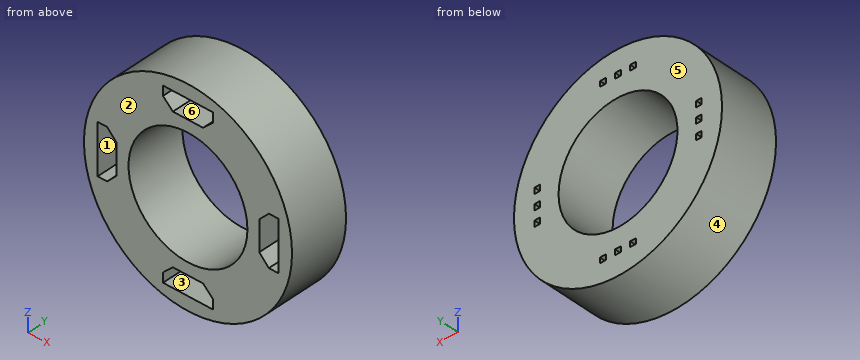
from build123d import *

# Parameters (mm, degrees)
F0_R     = 8.75
F0_R_2   = 5
F1_DEPTH = 5
F0_W     = 0.5
F0_H     = 0.45
F0_W_2   = 0.45
F0_H_2   = 0.5
F2_DEPTH = 1.5


with BuildPart() as f1:
    # F0 (on Front) → F1 (new body)
    with BuildSketch(Plane.XZ):
        Circle(F0_R)
        Polygon((-2.1, -6.8), (-1.27, -6), (1.27, -6), (2.1, -6.8), (2.1, -7.6), (-2.1, -7.6), align=None, mode=Mode.SUBTRACT)
        Polygon((-6.8, 2.1), (-6, 1.27), (-6, -1.27), (-6.8, -2.1), (-7.6, -2.1), (-7.6, 2.1), align=None, mode=Mode.SUBTRACT)
        Circle(F0_R_2, mode=Mode.SUBTRACT)
        Polygon((6.8, -2.1), (6, -1.27), (6, 1.27), (6.8, 2.1), (7.6, 2.1), (7.6, -2.1), align=None, mode=Mode.SUBTRACT)
        Polygon((-2.1, 6.8), (-2.1, 7.6), (2.1, 7.6), (2.1, 6.8), (1.27, 6), (-1.27, 6), align=None, mode=Mode.SUBTRACT)
    extrude(amount=F1_DEPTH)

    # F0 (on Front) → F2 (join)
    with BuildSketch(Plane.XZ):
        Polygon((2.1, 7.6), (-2.1, 7.6), (-2.1, 6.8), (-1.27, 6), (1.27, 6), (2.1, 6.8), align=None)
        with Locations((-1.27, 6.8)):
            Rectangle(F0_W, F0_H, mode=Mode.SUBTRACT)
        with Locations((0, 6.8)):
            Rectangle(F0_W, F0_H, mode=Mode.SUBTRACT)
        with Locations((1.27, 6.8)):
            Rectangle(F0_W, F0_H, mode=Mode.SUBTRACT)
        Polygon((-6, -1.27), (-6, 1.27), (-6.8, 2.1), (-7.6, 2.1), (-7.6, -2.1), (-6.8, -2.1), align=None)
        with Locations((-6.8, -1.27)):
            Rectangle(F0_W_2, F0_H_2, mode=Mode.SUBTRACT)
        with Locations((-6.8, 0)):
            Rectangle(F0_W_2, F0_H_2, mode=Mode.SUBTRACT)
        with Locations((-6.8, 1.27)):
            Rectangle(F0_W_2, F0_H_2, mode=Mode.SUBTRACT)
        Polygon((1.27, -6), (-1.27, -6), (-2.1, -6.8), (-2.1, -7.6), (2.1, -7.6), (2.1, -6.8), align=None)
        with Locations((-1.27, -6.8)):
            Rectangle(F0_W, F0_H, mode=Mode.SUBTRACT)
        with Locations((0, -6.8)):
            Rectangle(F0_W, F0_H, mode=Mode.SUBTRACT)
        with Locations((1.27, -6.8)):
            Rectangle(F0_W, F0_H, mode=Mode.SUBTRACT)
        Polygon((6, 1.27), (6, -1.27), (6.8, -2.1), (7.6, -2.1), (7.6, 2.1), (6.8, 2.1), align=None)
        with Locations((6.8, -1.27)):
            Rectangle(F0_W_2, F0_H_2, mode=Mode.SUBTRACT)
        with Locations((6.8, 0)):
            Rectangle(F0_W_2, F0_H_2, mode=Mode.SUBTRACT)
        with Locations((6.8, 1.27)):
            Rectangle(F0_W_2, F0_H_2, mode=Mode.SUBTRACT)
    extrude(amount=F2_DEPTH)


solid = f1.part
Check sheet for the modelled part. Datum: model origin and axes. Units: mm. Face numbers are marked on the shaded views. A direction names the side the tool comes from. Coordinates: 2 decimals unless noted, no trailing zeros. Loops run counter-clockwise (first coordinate to the right, second up) from the corner with the lowest first, then second, coordinate; pieces in that order, holes last. Notation, with made-up numbers: (77.5, 56.25) -> (125.5, 56.25) arc R22 cw to (125.5, 71.25) -> close; hole circle Ø9 at (12, -31). An arc over 180 degrees is marked (long way). Answer in a Markdown table with one row per item.
1. Sectioned sample at C-C, the plane y = -2.05. Record the boundary of the cut face in (x, z), then the cut area to 3 significant figures.
Check values:
| item | result |
|---|---|
| outline | circle Ø17.5 at (0, 0); hole (-7.6, -2.1) -> (-6.8, -2.1) -> (-6, -1.27) -> (-6, 1.27) -> (-6.8, 2.1) -> (-7.6, 2.1) -> close; hole circle Ø10 at (0, 0); hole (-2.1, -7.6) -> (2.1, -7.6) -> (2.1, -6.8) -> (1.27, -6) -> (-1.27, -6) -> (-2.1, -6.8) -> close; hole (-2.1, 6.8) -> (-1.27, 6) -> (1.27, 6) -> (2.1, 6.8) -> (2.1, 7.6) -> (-2.1, 7.6) -> close; hole (6, -1.27) -> (6.8, -2.1) -> (7.6, -2.1) -> (7.6, 2.1) -> (6.8, 2.1) -> (6, 1.27) -> close |
| area | 138 mm2 |
2. Go/stop test with flat-tipped pins: pin 1 (2 mm diameter, centred on x = -2.5, y = -1, fed in from -Z); pin 2 (0.6 mm diameter, centred on y = -3.5, z = 7, fed in from +X); pin 3 (0.6 mm diameter, centred on x = 1.5, y = -1, fed in from -Z). Record where each tip stops, or that it passes through.
Check values:
| item | result |
|---|---|
| pin 1 | stops at z = -8.62 |
| pin 2 | stops at x = 5.63 |
| pin 3 | stops at z = -8.67 |
3. Material ranges on line 1 along Z through (x, y) = (0, -2.1); line 2 along X through (y, z) = (-2.15, 2); line 3 along Z through (x, y) = (0, -1.45) (3 decimals), recorded low to high. Write a range as [from, to].
Check values:
| item | result |
|---|---|
| line 1 | z = [-8.75, -7.6], [-6, -5], [5, 6], [7.6, 8.75] |
| line 2 | x = [-8.52, -7.6], [-6.7, -4.58], [4.58, 6.7], [7.6, 8.52] |
| line 3 | z = [-8.75, -7.025], [-6.575, -5], [5, 6.575], [7.025, 8.75] |
4. Sectioned sample at B-B, the plane x = 0. Record the boundary of the cut face in (y, z) (3 decimals).
Check values:
| item | result |
|---|---|
| outline | (-5, -8.75) -> (0, -8.75) -> (0, -7.025) -> (-1.5, -7.025) -> (-1.5, -7.6) -> (-5, -7.6) -> close; (-5, -6) -> (-1.5, -6) -> (-1.5, -6.575) -> (0, -6.575) -> (0, -5) -> (-5, -5) -> close; (-5, 5) -> (0, 5) -> (0, 6.575) -> (-1.5, 6.575) -> (-1.5, 6) -> (-5, 6) -> close; (-5, 7.6) -> (-1.5, 7.6) -> (-1.5, 7.025) -> (0, 7.025) -> (0, 8.75) -> (-5, 8.75) -> close |
5. Release check for a two-part mould opening along X. For the marked faces 1, 2, 3 and 4 record: released by +X, released by -X, zero draft, split by the parting line, or undercut.
Check values:
| item | result |
|---|---|
| face 1 | undercut |
| face 2 | zero draft |
| face 3 | undercut |
| face 4 | split by the parting line |
6. Sectioned sample at D-D, the plane x = -3.5. Record the boundary of the cut face in (y, z), then the cut area to 3 significant figures.
Check values:
| item | result |
|---|---|
| outline | (-5, -8.02) -> (0, -8.02) -> (0, -3.57) -> (-5, -3.57) -> close; (-5, 3.57) -> (0, 3.57) -> (0, 8.02) -> (-5, 8.02) -> close |
| area | 44.5 mm2 |
7. Sectioned sample at A-A, the plane z = 0. Record the boundary of the cut face in (x, y) (3 decimals), then the cut area to 4 significant figures.
Check values:
| item | result |
|---|---|
| outline | (-8.75, -5) -> (-7.6, -5) -> (-7.6, -1.5) -> (-7.025, -1.5) -> (-7.025, 0) -> (-8.75, 0) -> close; (-6.575, -1.5) -> (-6, -1.5) -> (-6, -5) -> (-5, -5) -> (-5, 0) -> (-6.575, 0) -> close; (5, -5) -> (6, -5) -> (6, -1.5) -> (6.575, -1.5) -> (6.575, 0) -> (5, 0) -> close; (7.025, -1.5) -> (7.6, -1.5) -> (7.6, -5) -> (8.75, -5) -> (8.75, 0) -> (7.025, 0) -> close |
| area | 24.95 mm2 |
8. Access from +Z, -Z, +X, -X, +Y, -Y to the whole of each face (thin tool, end or side, straight path). Record for the marked faces 5 and 6.
Check values:
| item | result |
|---|---|
| face 5 | +Z, -Z, +X, -X, +Y |
| face 6 | -Y |
